Geometry: final body of the model. Coordinates: model frame, mm. Face numbers are marked on the shaded views. A direction names the side the tool comes from. Give positions to 0.01 mm unless a question says otherwise; leave off trailing zeros. Loops run counter-clockwise (first coordinate to the right, second up) from the corner with the lowest first, then second, coordinate; pieces in that order, holes last. Notation, with made-up numbers: (-33, 15.5) - (-20, 15.5) arc R19 cw to (-20, 23.5) - close; hole circle Ø2 at (69, 33.25). An arc over 180 degrees is marked (long way). Answer in a Markdown table with one row per item.
from build123d import *

# Parameters (mm, degrees)
EXTRUDE_1_DEPTH          = 80
EXTRUDE_1_DEPTH_BACK     = 5
SKETCH_2_R               = 12
SKETCH_1_R               = 2
CUT_EXTRUDE_1_DEPTH      = 80
SKETCH_4_R               = 15
EXTRUDE_2_DEPTH          = 2
CUT_EXTRUDE_START        = -40
CUT_EXTRUDE_2_DEPTH      = 40
CUT_EXTRUDE_3_DEPTH      = 40
CUT_EXTRUDE_3_DEPTH_BACK = 40
SKETCH_8_R               = 2
SKETCH_10_R              = 1
CUT_EXTRUDE_4_DEPTH      = 83.764726883


with BuildPart() as part:
    # 草图2 → 凸台-拉伸1 (new, two sides: drawn at the far end of the back side and taken through both)
    with BuildSketch(Plane(origin=(0, 0, 0), x_dir=(0, 0, -1), z_dir=(1, 0, 0)).offset(-EXTRUDE_1_DEPTH_BACK)):
        Circle(SKETCH_2_R)
    extrude(amount=EXTRUDE_1_DEPTH + EXTRUDE_1_DEPTH_BACK)

    # 草图1 → 切除-拉伸1 (cut)
    with BuildSketch(Plane(origin=(0, 0, 0), x_dir=(1, 0, 0), z_dir=(0, 1, 0))):
        with Locations(Location((0, 0, 0), (0, 0, 270))):
            Circle(SKETCH_1_R)
    extrude(amount=-CUT_EXTRUDE_1_DEPTH, mode=Mode.SUBTRACT)

    # 草图4 → 凸台-拉伸2 (add)
    with BuildSketch(Plane(origin=(5, 0, 0), x_dir=(0, 0, -1), z_dir=(1, 0, 0))):
        Circle(SKETCH_4_R)
    extrude(amount=-EXTRUDE_2_DEPTH)

    # 草图7 → 切除-拉伸2 (cut)
    with BuildSketch(Plane(origin=(80, 0, 0), x_dir=(0, 0, -1), z_dir=(1, 0, 0)).offset(CUT_EXTRUDE_START)):
        with BuildLine():
            ThreePointArc((2, 11.832159566), (0, 12), (-2, 11.832159566))
            Line((-2, 11.832159566), (-2, -11.832159566))
            ThreePointArc((-2, -11.832159566), (0, -12), (2, -11.832159566))
            Line((2, -11.832159566), (2, 11.832159566))
        make_face()
    extrude(amount=CUT_EXTRUDE_2_DEPTH, mode=Mode.SUBTRACT)

    # 草图8 → 切除-拉伸3 (cut, two sides: drawn at the far end of the back side and taken through both)
    with BuildSketch(Plane.XY.offset(-2).offset(-CUT_EXTRUDE_3_DEPTH_BACK)):
        with Locations(Location((70, 0, 0), (0, 0, 180))):
            Circle(SKETCH_8_R)
    extrude(amount=CUT_EXTRUDE_3_DEPTH + CUT_EXTRUDE_3_DEPTH_BACK, mode=Mode.SUBTRACT)

    # 草图10 → 切除-拉伸4 (cut, through all)
    with BuildSketch(Plane(origin=(0, 0, 0), x_dir=(0, 0, -1), z_dir=(1, 0, 0))):
        with Locations((0, -8)):
            Circle(SKETCH_10_R)
    extrude(amount=-CUT_EXTRUDE_4_DEPTH, mode=Mode.SUBTRACT)


solid = part.part
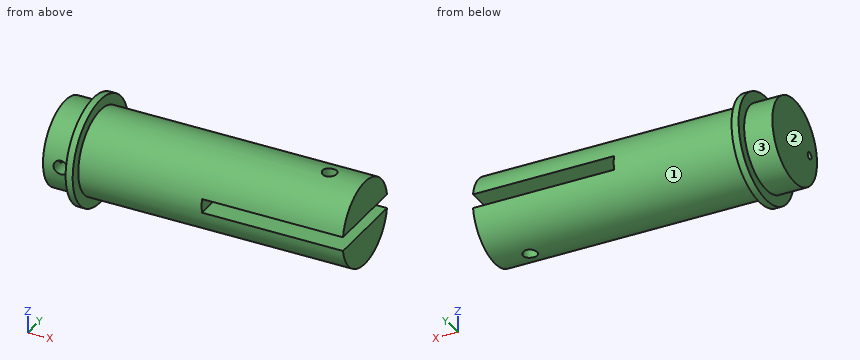
Q1. Cut plane B-B (x = 70). Output: boundary loops of the cut face in (y, z), and give its area (3 significant figures).
Check values:
| item | result |
|---|---|
| outline | (-11.83, -2) arc R12 ccw to (-2, -11.83) - (-2, -2) - close; (-11.83, 2) - (-2, 2) - (-2, 11.83) arc R12 ccw to start; (2, -11.83) arc R12 ccw to (11.83, -2) - (2, -2) - close; (2, 2) - (11.83, 2) arc R12 ccw to (2, 11.83) - close |
| area | 277 mm² |
Q2. Material intervals for line 1 along X through (y, z) = (-6.75, 0); line 2 along X through (y, z) = (-7.25, 9.75); line 3 along Z through (x, y) = (73.5, 2.5), sorted ascending.
Check values:
| item | result |
|---|---|
| line 1 | -5 to -2, 2 to 40 |
| line 2 | 3 to 5 |
| line 3 | -11.74 to -2, 2 to 11.74 |
Q3. Cut plane A-A (z = 0). Output: boundary loops of the cut face in (x, y), and give its area (3 significant figures).
Check values:
| item | result |
|---|---|
| outline | (-5, -12) - (-2, -12) - (-2, -9) - (-5, -9) - close; (-5, -7) - (-2, -7) - (-2, 0) - (2, 0) - (2, -12) - (3, -12) - (3, -15) - (5, -15) - (5, -12) - (40, -12) - (40, 12) - (5, 12) - (5, 15) - (3, 15) - (3, 12) - (-5, 12) - close |
| area | 1,040 mm² |
Q4. Cut plane D-D (z = -8). Output: boundary loops of the cut face in (x, y).
Check values:
| item | result |
|---|---|
| outline | (-5, -8.94) - (3, -8.94) - (3, -12.69) - (5, -12.69) - (5, -8.94) - (80, -8.94) - (80, 8.94) - (5, 8.94) - (5, 12.69) - (3, 12.69) - (3, 8.94) - (-5, 8.94) - close; hole circle Ø4 at (70, 0) |
Q5. Reachability of the marked faces 1, 2 and 3 from +Z, -Z, +X, -X, +Y, -Y: full face, straight path, thin tool, end or side. Return the list, or none.
Check values:
| item | result |
|---|---|
| face 1 | +X |
| face 2 | +Z, -Z, -X, +Y, -Y |
| face 3 | -X |
Q6. Cut plane C-C (y = -3). Output: boundary loops of the cut face in (x, z), and give its area (3 significant figures).
Check values:
| item | result |
|---|---|
| outline | (-5, -11.62) - (3, -11.62) - (3, -14.7) - (5, -14.7) - (5, -11.62) - (80, -11.62) - (80, -2) - (40, -2) - (40, 2) - (80, 2) - (80, 11.62) - (5, 11.62) - (5, 14.7) - (3, 14.7) - (3, 11.62) - (-5, 11.62) - close; hole circle Ø4 at (0, 0) |
| area | 1,810 mm² |
Q7. First-contact query: pin 1 (3 mm diameter, centred on x = 25.5, y = -11.5, fed in from -Z); pin 2 (4 mm diameter, centred on x = 38, y = -1, fed in from +Z); pin 3 (2 mm diameter, centred on y = 4, z = 0.5, fed in from +X). Flat tips, straight axial feed; report the tip coordinate or a pass-through.
Check values:
| item | result |
|---|---|
| pin 1 | z = -6.63 |
| pin 2 | z = 12 |
| pin 3 | x = 40 |
